Model file for the job. Use its own axes, mm. Face numbers are marked on the shaded views. A direction names the side the tool comes from. Give positions to 0.01 mm unless a question says otherwise; leave off trailing zeros. Write each loop counter-clockwise with the first axis right and the second up, starting at its lowest first coordinate (ties: lowest second). Pieces come first, ordered by that corner, then holes. Notation, with made-up numbers: (58.5, 35) - (83.5, 35) arc R18 cw to (83.5, 65) - close; hole circle Ø4 at (42, 53.5). An arc over 180 degrees is marked (long way). One line per item, written item: value. Start each with the question number.
(1) Cut at B-B, the plane z = 0. List the corners of the cut face in (x, y).
(2) Drop flat-ended pins along their axis: P1, Ø5, axis at x = -11.5, y = 8, coming from the +Z side; P2, Ø12, axis at y = 13.5, z = 27.5, coming from the -X side; P3, Ø8, axis at x = 62.5, z = -2, coming from the +Y side; P4, Ø5, axis at y = 17, z = 3, coming from the +X side. Give the stop position or say it passes through.
(3) Cut at C-C, the plane z = 62.8. List the corners of the cut face in (x, y).
(4) Cut at A-A, the plane x = -59.8. List the corners of the cut face in (y, z).
(5) 3-axis set-ups, long thin cutter, end or side, ignore diameter. For the marked faces 1, 2, 3, 4 and 5: which of +Z, -Z, +X, -X, +Y, -Y reach the whole face in a straight line?
(6) Cut at D-D, the plane y = 6.5. List the corners of the cut face in (x, z).
(7) Probe L1, parallel to X at y = 4.75, z = 0; L2, parallel to X at y = 5.25, z = 62.8; L3, parallel to Z at x = -59.8, y = 2. List the from-to ranges inside material, lowest first.
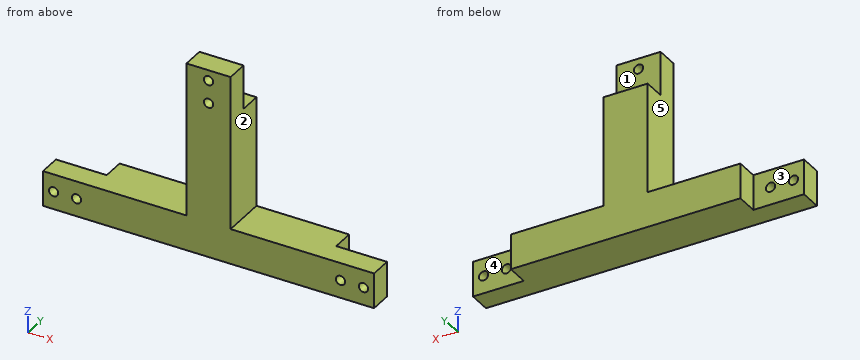
from build123d import *

# Parameters (mm, degrees)
SKETCH_1_W          = 150
SKETCH_1_H          = 16
EXTRUDE_1_DEPTH     = 10
SKETCH_2_W          = 110
SKETCH_2_H          = 16
EXTRUDE_2_DEPTH     = 10
SKETCH_4_R          = 2.1
CUT_EXTRUDE_1_DEPTH = 10
SKETCH_5_R          = 2.1
CUT_EXTRUDE_2_DEPTH = 10
SKETCH_6_W          = 20
SKETCH_6_H          = 20
EXTRUDE_3_DEPTH     = 50
SKETCH_7_W          = 20
SKETCH_7_H          = 10
EXTRUDE_4_DEPTH     = 20
SKETCH_8_R          = 2.1
CUT_EXTRUDE_3_DEPTH = 10
SKETCH_9_W          = 3
SKETCH_9_H          = 16
CUT_EXTRUDE_4_DEPTH = 10


with BuildPart() as part:
    # 草图1 → 凸台-拉伸1 (new body)
    with BuildSketch(Plane(origin=(0, 0, 0), x_dir=(1, 0, 0), z_dir=(0, 1, 0))):
        Rectangle(SKETCH_1_W, SKETCH_1_H)
    extrude(amount=EXTRUDE_1_DEPTH)

    # 草图2 → 凸台-拉伸2 (add)
    with BuildSketch(Plane(origin=(0, 10, 0), x_dir=(1, 0, 0), z_dir=(0, 1, 0))):
        Rectangle(SKETCH_2_W, SKETCH_2_H)
    extrude(amount=EXTRUDE_2_DEPTH)

    # 草图4 → 切除-拉伸1 (cut)
    with BuildSketch(Plane(origin=(0, 10, 0), x_dir=(1, 0, 0), z_dir=(0, 1, 0))):
        with Locations((-70.2, 0)):
            Circle(SKETCH_4_R)
        with Locations((-59.8, 0)):
            Circle(SKETCH_4_R)
    extrude(amount=-CUT_EXTRUDE_1_DEPTH, mode=Mode.SUBTRACT)

    # 草图5 → 切除-拉伸2 (cut)
    with BuildSketch(Plane(origin=(0, 10, 0), x_dir=(1, 0, 0), z_dir=(0, 1, 0))):
        with Locations((59.8, 0)):
            Circle(SKETCH_5_R)
        with Locations((70.2, 0)):
            Circle(SKETCH_5_R)
    extrude(amount=-CUT_EXTRUDE_2_DEPTH, mode=Mode.SUBTRACT)

    # 草图6 → 凸台-拉伸3 (add)
    with BuildSketch(Plane.XY.offset(8)):
        with Locations((0, 10)):
            Rectangle(SKETCH_6_W, SKETCH_6_H)
    extrude(amount=EXTRUDE_3_DEPTH)

    # 草图7 → 凸台-拉伸4 (add)
    with BuildSketch(Plane.XY.offset(58)):
        with Locations((0, 5)):
            Rectangle(SKETCH_7_W, SKETCH_7_H)
    extrude(amount=EXTRUDE_4_DEPTH)

    # 草图8 → 切除-拉伸3 (cut)
    with BuildSketch(Plane(origin=(0, 10, 0), x_dir=(1, 0, 0), z_dir=(0, 1, 0))):
        with Locations((0, -62.8)):
            Circle(SKETCH_8_R)
        with Locations((0, -73.2)):
            Circle(SKETCH_8_R)
    extrude(amount=-CUT_EXTRUDE_3_DEPTH, mode=Mode.SUBTRACT)

    # 草图9 → 切除-拉伸4 (cut)
    with BuildSketch(Plane(origin=(0, 20, 0), x_dir=(1, 0, 0), z_dir=(0, 1, 0))):
        with Locations((-53.5, 0)):
            Rectangle(SKETCH_9_W, SKETCH_9_H)
        with Locations((53.5, 0)):
            Rectangle(SKETCH_9_W, SKETCH_9_H)
    extrude(amount=-CUT_EXTRUDE_4_DEPTH, mode=Mode.SUBTRACT)


solid = part.part
Answers follow:
1. outline: (-75, 0) - (-72.3, 0) - (-72.3, 10) - (-75, 10) - close; (-68.1, 0) - (-61.9, 0) - (-61.9, 10) - (-68.1, 10) - close; (-57.7, 0) - (57.7, 0) - (57.7, 10) - (52, 10) - (52, 20) - (-52, 20) - (-52, 10) - (-57.7, 10) - close; (61.9, 0) - (68.1, 0) - (68.1, 10) - (61.9, 10) - close; (72.3, 0) - (75, 0) - (75, 10) - (72.3, 10) - close
2. P1: stops at z = 78
2. P2: stops at x = -10
2. P3: stops at y = 10
2. P4: stops at x = 52
3. outline: (-10, 0) - (-2.1, 0) - (-2.1, 10) - (-10, 10) - close; (2.1, 0) - (10, 0) - (10, 10) - (2.1, 10) - close
4. outline: (0, -8) - (10, -8) - (10, -2.1) - (0, -2.1) - close; (0, 2.1) - (10, 2.1) - (10, 8) - (0, 8) - close
5. face 1: +Z, +X, -X, +Y
5. face 2: +Z, +X, +Y, -Y
5. face 3: +Z, -Z, -X, +Y
5. face 4: +Z, -Z, +X, +Y
5. face 5: +Z, -X, +Y, -Y
6. outline: (-75, -8) - (75, -8) - (75, 8) - (10, 8) - (10, 78) - (-10, 78) - (-10, 8) - (-75, 8) - close; hole circle Ø4.2 at (-70.2, 0); hole circle Ø4.2 at (-59.8, 0); hole circle Ø4.2 at (0, 62.8); hole circle Ø4.2 at (0, 73.2); hole circle Ø4.2 at (59.8, 0); hole circle Ø4.2 at (70.2, 0)
7. L1: x = -75 to -72.3, -68.1 to -61.9, -57.7 to 57.7, 61.9 to 68.1, 72.3 to 75
7. L2: x = -10 to -2.1, 2.1 to 10
7. L3: z = -8 to -2.1, 2.1 to 8
